Autodesk Inventor part; units mm, degrees
ref_plane "YZ Plane" through (0, 0, 0) normal (1, 0, 0) x (0, 1, 0)
ref_plane "XZ Plane" through (0, 0, 0) normal (0, 1, 0) x (-1, 0, 0)
ref_plane "XY Plane" through (0, 0, 0) normal (0, 0, 1) x (1, 0, 0)
sketch "Sketch1" plane through (0, 0, 0) normal (0, 1, 0) x (-1, 0, 0)
  circle A0 centre (0, 0) radius 27.305
  dimension "d85" = 54.61
extrude "Extrusion1" add sketch "Sketch1" along normal blind 3.175
sketch "Sketch2" plane through (0, 3.175, 0) normal (0, 1, 0) x (1, 0, 0)
  circle A0 centre (0, -22.86) radius 1.905
  circle A1 centre (0, 22.86) radius 1.905
  circle A2 centre (0, 0) radius 3.4925
  circle A3 centre (0, 0) radius 27.305
  line L0 (0, 0) -> (0, -35.2816) construction
  line L1 (0, 0) -> (-33.3398, 0) construction
  circle A4 centre (0, -22.86) radius 4.7625
  dimension "d105" = 6.985
  dimension "d107" = 3.81
  dimension "d109" = 3.81
  dimension "d147" = 0
  dimension "d148" = 0
  dimension "d149" = 22.86
  dimension "d150" = 22.86
  dimension "d151" = 9.525
sketch "Sketch3" plane through (0, 0, 0) normal (0, -1, 0) x (1, 0, 0)
  line L0 (-12.7, -4.445) -> (-2.54, -4.445)
  line L1 (-2.54, -4.445) -> (-2.54, 4.445)
  line L2 (-2.54, 4.445) -> (-12.7, 4.445)
  line L3 (-12.7, 4.445) -> (-12.7, -4.445)
  line L4 (-38.227, 0) -> (38.227, 0)
  line L5 (0, -38.227) -> (0, 38.227)
  point P0 (0, 0)
  dimension "d116" = 10.16
  dimension "d125" = 8.89
  dimension "d126" = 12.7
extrude "Extrusion3" [suppressed]
fillet "Fillet1" [suppressed]
sketch "Sketch4" plane through (0, 3.175, 0) normal (0, 1, 0) x (1, 0, 0)
  circle A0 centre (0, 0) radius 27.305
  line L0 (-7.62, -26.2202) -> (-7.62, 26.2202)
  line L1 (19.05, -19.5617) -> (19.05, 19.5617)
  dimension "d121" = 7.62
  dimension "d122" = 19.05
extrude "Extrusion4" cut sketch "Sketch4" against normal through all contours A0 L1 | L0 A0
hole "Hole10" at (0, 3.175, -22.86) at (0, 3.175, 22.86) direction (0, -1, 0) diameter 2.6416 end through all
sketch "Sketch5" plane through (0, 3.175, 0) normal (0, 1, 0) x (1, 0, 0)
  line L0 (0, 0) -> (23.5566, 0) construction
  line L1 (19.05, -19.5617) -> (19.05, 19.5617)
  point P0 (8.89, 12.6873)
  point P1 (8.89, -12.6873)
  point P2 (-3.81, -12.6873)
  point P3 (-3.81, 12.6873)
  dimension "d136" = 25.3746
  dimension "d137" = 12.7
  dimension "d146" = 22.86
  dimension "d160" = 22.86
  dimension "d161" = 10.16
hole "Hole11" at (8.89, 3.175, -12.6873) at (8.89, 3.175, 12.6873) at (-3.81, 3.175, 12.6873) at (-3.81, 3.175, -12.6873) direction (0, -1, 0) diameter 3.81 depth 25.4 tip angle 118
sketch "Sketch6" plane through (0, 0, 0) normal (0, -1, 0) x (1, 0, 0)
  circle A0 centre (8.1279, 0.0315) radius 1.5875
  circle A1 centre (6.5218, 4.8509) radius 1.5875
  circle A2 centre (8.1279, 0.0315) radius 1.5875
  line L0 (-0.8446, 5.1702) -> (-2.5619, 10.3231)
  arc A3 (4.1433, -9.7961) -> (-2.5619, 10.3231) centre (0, 0) ccw
  line L1 (4.1433, -9.7961) -> (2.426, -4.6432)
  arc A4 (2.426, -4.6432) -> (-0.8446, 5.1702) centre (0, 0) ccw
  point P0 (0, 0)
hole "Hole12" at (8.1279, 0, 0.0315) at (6.5218, 0, 4.8509) direction (0, 1, 0) diameter 3.175 end through all
fillet "Fillet2" radius 3.175 4 edges at (-7.62, 1.5875, 26.2202) (-7.62, 1.5875, -26.2202) (19.05, 1.5875, 19.5617) (19.05, 1.5875, -19.5617)
equation "\"d107\" = d106"
equation "\"d109\" = d106"
equation "\"d150\" = d149"
properties part number "Shield_3_Ground_v4" material "Stainless Steel"
For this review, take the finished solid that the model builds, in its own axes (mm). Round coordinates to 2 decimals unless told otherwise and drop trailing zeros. Write each loop counter-clockwise with the first axis right and the second up, starting at its lowest first coordinate (ties: lowest second). Pieces come first, ordered by that corner, then holes. Notation, with made-up numbers: (3, 59) - (35, 59) arc R23 cw to (35, 91) - close; hole circle Ø7 at (20.25, 77). An arc over 180 degrees is marked (long way). Write item = value, one per line. Start each with the question number.
1. Consider section B-B on z = 4.5. State the section outline as (x, y) points (3 decimals), plus the area to 3 significant figures.
2. Draft analysis for pull direction X (two halves, no side actions). For faces 1 (the face through (7.021, 1.565, -26.387)), 2 (the face through (6, 3.175, 0)), 3 (the face through (8.806, 1.565, 10.784)), state which applies: released by +X, released by -X, zero draft, split by the parting line, or undercut.
3. Consider section C-C on x = 8.89. State the section outline as (y, z) points (3 decimals), plus the area to 3 significant figures.
4. Wall thickness on L1, parallel to Z at x = -2.5, y = 0.75; L2, parallel to Z at x = -3.5, y = 1.7; L3, parallel to Z at x = 7.75, y = 2.4: over which ranges is each line inside the solid? List them lowest first.
5. Consider section A-A on x = 0. State the section outline as (y, z) points (3 decimals), plus the area to 3 significant figures.
6. Consider section D-D on y = 2.55. Give the number of separate pieces and of enclosed holes in the cut face, plus the area to 3 significant figures.
Evaluation:
q1.outline = (-7.62, 0) - (4.974, 0) - (4.974, 3.175) - (-7.62, 3.175) - close; (8.07, 0) - (19.05, 0) - (19.05, 3.175) - (8.07, 3.175) - close
q1.area = 74.8 mm2
q2.face_1 = split by the parting line
q2.face_2 = zero draft
q2.face_3 = undercut
q3.outline = (0, -25.817) - (3.175, -25.817) - (3.175, -14.592) - (0, -14.592) - close; (0, -10.782) - (3.175, -10.782) - (3.175, -1.361) - (0, -1.361) - close; (0, 1.424) - (3.175, 1.424) - (3.175, 10.782) - (0, 10.782) - close; (0, 14.592) - (3.175, 14.592) - (3.175, 25.817) - (0, 25.817) - close
q3.area = 131 mm2
q4.L1 = -27.19 to -14.07, -11.3 to 11.3, 14.07 to 27.19
q4.L2 = -27.08 to -14.57, -10.81 to 10.81, 14.57 to 27.08
q4.L3 = -26.18 to -14.21, -11.16 to -1.51, 1.57 to 3.85, 5.86 to 11.16, 14.21 to 26.18
q5.outline = (0, -27.305) - (3.175, -27.305) - (3.175, -24.181) - (0, -24.181) - close; (0, -21.539) - (3.175, -21.539) - (3.175, 21.539) - (0, 21.539) - close; (0, 24.181) - (3.175, 24.181) - (3.175, 27.305) - (0, 27.305) - close
q5.area = 157 mm2
q6.separate_pieces = 1
q6.enclosed_holes = 8
q6.area = 1,280 mm2
